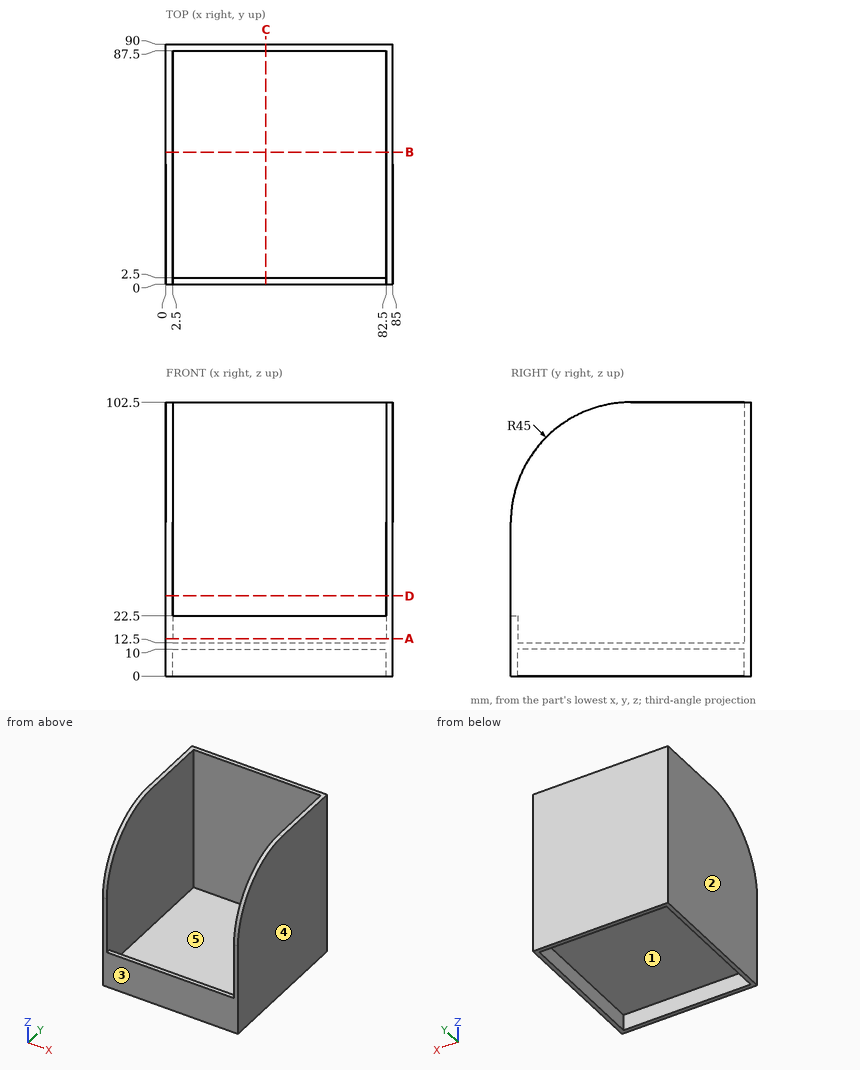
Answer from the drawing. Dimensions are ordinates in mm from the lowest x, y and z of the part. A direction names the side the tool comes from. Round coordinates to 2 decimals unless told otherwise and drop trailing zeros. Loops run counter-clockwise (first coordinate to the right, second up) from the corner with the lowest first, then second, coordinate; pieces in that order, holes last.
Q1. Which of the six approach directions +Z, -Z, +X, -X, +Y, -Y give full straight-line access (tool end or side, diameter ignored) to the marked faces 4 and 5?
Q2. Section B-B on y = 49.5 is taken. Write down the section's boundary in (x, z), and give its area (4 significant figures).
Q3. Consider probe 1 along X at (y, z) = (35.5, 40); probe 2 along Y at (x, z) = (76.5, 21); probe 3 along Y at (x, z) = (60.5, 34). Determine where each line is inside the solid, lowest interval first.
Q4. Determine the mould class of the marked faces 1, 2 and 3 for opening direction X: released by +X, released by -X, zero draft, split by the parting line, or undercut.
Q5. Section C-C on x = 37.5 is taken. Write down the section's boundary in (y, z).
Q6. Section D-D on z = 30 is taken. Write down the section's boundary in (x, y).
Q7. Each of these flat-tipped pins is pushed along its axis until it touches: pin 1 (5 mm diameter, centred on x = 25, y = 30.5, fed in from +Z); pin 2 (12 mm diameter, centred on x = 28, y = 80, fed in from -Z); pin 3 (2 mm diameter, centred on x = 24.5, y = 1, fed in from +Z). Where does it stop, or does it pass through?
Q8. Section A-A on z = 14 is taken. Write down the section's boundary in (x, y), and give its area (3 significant figures).
Output:
1. face 4: +Z, -Z, +X, +Y, -Y
1. face 5: +Z
2. outline: (0, 0) - (2.5, 0) - (2.5, 10) - (82.5, 10) - (82.5, 0) - (85, 0) - (85, 102.5) - (82.5, 102.5) - (82.5, 12.5) - (2.5, 12.5) - (2.5, 102.5) - (0, 102.5) - close
2. area: 712.5 mm2
3. probe 1: x = 0 to 2.5, 82.5 to 85
3. probe 2: y = 0 to 2.5, 87.5 to 90
3. probe 3: y = 87.5 to 90
4. face 1: undercut
4. face 2: released by -X
4. face 3: zero draft
5. outline: (0, 0) - (2.5, 0) - (2.5, 10) - (87.5, 10) - (87.5, 0) - (90, 0) - (90, 102.5) - (87.5, 102.5) - (87.5, 12.5) - (2.5, 12.5) - (2.5, 22.5) - (0, 22.5) - close
6. outline: (0, 0) - (2.5, 0) - (2.5, 87.5) - (82.5, 87.5) - (82.5, 0) - (85, 0) - (85, 90) - (0, 90) - close
7. pin 1: stops at z = 12.5
7. pin 2: stops at z = 10
7. pin 3: stops at z = 22.5
8. outline: (0, 0) - (85, 0) - (85, 90) - (0, 90) - close; hole (2.5, 2.5) - (82.5, 2.5) - (82.5, 87.5) - (2.5, 87.5) - close
8. area: 850 mm2
